from build123d import *

# Parameters (mm, degrees)
IZIM1_W                     = 28
IZIM1_H                     = 28
Y_KSEKLIK_EKSTR_ZYON1_DEPTH = 585
IZIM2_R                     = 6
KES_EKSTR_ZYON1_DEPTH       = 60
SKETCH1_R                   = 3.5
CUT_EXTRUDE1_DEPTH          = 25
SKETCH3_R                   = 3
CUT_EXTRUDE2_DEPTH          = 586.837008049
SKETCH5_R                   = 4.25
CUT_EXTRUDE4_DEPTH          = 6
SKETCH6_W                   = 68.791406121
SKETCH6_H                   = 219.206637727
SKETCH6_W_2                 = 68.987868966
SKETCH6_H_2                 = 174.940464565
CUT_EXTRUDE5_DEPTH          = 0.3
SKETCH7_R                   = 3
CUT_EXTRUDE6_DEPTH          = 84
SKETCH8_R                   = 5
CUT_EXTRUDE7_DEPTH          = 6


with BuildPart() as part:
    # Çizim1 → Yükseklik-Ekstrüzyon1 (new body)
    with BuildSketch(Plane.XY):
        Rectangle(IZIM1_W, IZIM1_H)
    extrude(amount=Y_KSEKLIK_EKSTR_ZYON1_DEPTH)

    # Çizim2 → Kes-Ekstrüzyon1 (cut)
    with BuildSketch(Plane.XY.offset(585)):
        Circle(IZIM2_R)
    extrude(amount=-KES_EKSTR_ZYON1_DEPTH, mode=Mode.SUBTRACT)

    # Sketch1 → Cut-Extrude1 (cut)
    with BuildSketch(Plane(origin=(0, 0, 0), x_dir=(-1, 0, 0), z_dir=(0, 0, -1))):
        with Locations((-7, 7)):
            Circle(SKETCH1_R)
        with Locations((7, -7)):
            Circle(SKETCH1_R)
    extrude(amount=-CUT_EXTRUDE1_DEPTH, mode=Mode.SUBTRACT)

    # Sketch3 → Cut-Extrude2 (cut, through all)
    with BuildSketch(Plane.ZY.offset(14)):
        with Locations((485, 0)):
            Circle(SKETCH3_R)
    extrude(amount=-CUT_EXTRUDE2_DEPTH, mode=Mode.SUBTRACT)

    # Sketch5 → Cut-Extrude4 (cut)
    with BuildSketch(Plane.ZY.offset(14)):
        with Locations((485, 0)):
            Circle(SKETCH5_R)
    extrude(amount=-CUT_EXTRUDE4_DEPTH, mode=Mode.SUBTRACT)

    # Sketch6 → Cut-Extrude5 (cut)
    with BuildSketch(Plane.ZY.offset(14)):
        with Locations((586.39570306, 18.878857334)):
            Rectangle(SKETCH6_W, SKETCH6_H)
        with Locations((25.006065517, 7.665656751)):
            Rectangle(SKETCH6_W_2, SKETCH6_H_2)
    extrude(amount=-CUT_EXTRUDE5_DEPTH, mode=Mode.SUBTRACT)

    # Sketch7 → Cut-Extrude6 (cut)
    with BuildSketch(Plane(origin=(14, 0, 0), x_dir=(0, 0, -1), z_dir=(1, 0, 0))):
        with Locations((-15, 0)):
            Circle(SKETCH7_R)
    extrude(amount=-CUT_EXTRUDE6_DEPTH, mode=Mode.SUBTRACT)

    # Sketch8 → Cut-Extrude7 (cut)
    with BuildSketch(Plane(origin=(14, 0, 0), x_dir=(0, 0, -1), z_dir=(1, 0, 0))):
        with Locations((-15, 0)):
            Circle(SKETCH8_R)
    extrude(amount=-CUT_EXTRUDE7_DEPTH, mode=Mode.SUBTRACT)


solid = part.part
Part model, mm, in its own coordinate system. A direction names the side the tool comes from. Coordinates: 2 decimals unless noted, no trailing zeros. Use a Markdown table: item, result. Add a question column.
Item 1: Which spindle directions (+Z, -Z, +X, -X, +Y, -Y) get a long thin tool onto all of the face, cutting with end or side? Do faces 5 (the flat face through (14, 0, 288)), 6 (the cylindrical face through (-6, 0, 555)). Say none if no direction does.
Item 2: Probe probe 1 along Y at (x, z) = (-12.4, 485); probe 2 along Z at (x, y) = (-0.5, -2); probe 3 along Z at (x, y) = (-9.75, -2.75). List the from-to ranges inside material, lowest first.
Item 3: Pull direction Y, two halves, no side cores. Call faces 1 (the cylindrical face through (11.04, -4.88, 16.08)), 2 (the flat face through (-13.7, 0, 29)), 3 (the flat face through (0, 0, 525)), 4 (the flat face through (0, 14, 288)): +Y half, -Y half, draft (parallel to the pull), parting line (faces both ways), or undercut.
Item 4: Flat gauge pins, fed straight in: P1, Ø9.5, axis at x = 0, y = 0, coming from the +Z side; P2, Ø3.5, axis at y = 0, z = 15, coming from the +X side; P3, Ø8, axis at y = 0, z = 15, coming from the +X side; P4, Ø14, axis at y = 7, z = 560.5, coming from the -X side. Where does each tip first touch, or does it go through?
Geometry says:
| question | item | result |
|---|---|---|
| 1 | face 5 | +Z, -Z, +X, +Y, -Y |
| 1 | face 6 | +Z |
| 2 | probe 1 | -14 to -4.25, 4.25 to 14 |
| 2 | probe 2 | 0 to 12.76, 17.24 to 482.76, 487.24 to 525 |
| 2 | probe 3 | 0 to 13.8, 16.2 to 481.76, 488.24 to 585 |
| 3 | face 1 | undercut |
| 3 | face 2 | draft |
| 3 | face 3 | undercut |
| 3 | face 4 | +Y half |
| 4 | P1 | z = 525 |
| 4 | P2 | through |
| 4 | P3 | x = 8 |
| 4 | P4 | x = -13.7 |
